from build123d import *

# Parameters (mm, degrees)
SKETCH1_W           = 70
SKETCH1_H           = 80
SKETCH1_R           = 17.5
SKETCH1_W_2         = 50
SKETCH1_H_2         = 30
BOSS_EXTRUDE1_DEPTH = 10
FILLET1_R           = 20
SKETCH2_R           = 2
CUT_EXTRUDE1_DEPTH  = 10


with BuildPart() as part:
    # Sketch1 → Boss-Extrude1 (new body)
    with BuildSketch(Plane.XY):
        with Locations((35, -40)):
            Rectangle(SKETCH1_W, SKETCH1_H)
        with Locations((35, -40)):
            Circle(SKETCH1_R, mode=Mode.SUBTRACT)
        with Locations((35, -95)):
            Rectangle(SKETCH1_W_2, SKETCH1_H_2)
    extrude(amount=BOSS_EXTRUDE1_DEPTH)

    # Fillet1
    fillet1_edges = [part.edges().sort_by_distance(p)[0] for p in [
        (70, 0, 5),
        (0, 0, 5),
    ]]
    fillet(fillet1_edges, radius=FILLET1_R)

    # Sketch2 → Cut-Extrude1 (cut)
    with BuildSketch(Plane.XY.offset(10)):
        with Locations((17.5, -22.5)):
            Circle(SKETCH2_R)
        with Locations((52.5, -22.5)):
            Circle(SKETCH2_R)
        with Locations((52.5, -57.5)):
            Circle(SKETCH2_R)
        with Locations((17.5, -57.5)):
            Circle(SKETCH2_R)
    extrude(amount=-CUT_EXTRUDE1_DEPTH, mode=Mode.SUBTRACT)


solid = part.part
CAD build for the part. Positions are in the model's coordinates, mm. A direction names the side the tool comes from. Round coordinates to 2 decimals unless told otherwise and drop trailing zeros. Write each loop counter-clockwise with the first axis right and the second up, starting at its lowest first coordinate (ties: lowest second). Pieces come first, ordered by that corner, then holes.
(1) 3-axis set-ups, long thin cutter, end or side, ignore diameter. For faces 5 (the face through (5, -80, 5)), 6 (the face through (52.24, -20.517, 5.07)), 7 (the face through (60, -95, 5)): which of +Z, -Z, +X, -X, +Y, -Y reach the whole face in a straight line?
(2) Slice it at D-D, the plane x = 62. Write the cut outline in (y, z).
(3) Mould opens along X. For faces 1 (the face through (17.24, -20.517, 5.07)), 2 (the face through (10, -95, 5)), 3 (the face through (64.297, -6.014, 5.07)), 4 (the face through (17.24, -55.517, 5.07)) say: pulls with the +X half, pulls with the -X half, needs draft (parallel to the pull), parting line crosses it, or undercut.
(4) Drop flat-ended pins along their axis: P1, Ø3.5, axis at x = 52.5, y = -22.5, coming from the -Z side; P2, Ø3, axis at x = 63.5, z = 3, coming from the -Y side. Give the stop position or say it passes through.
(5) Slice it at C-C, the plane z = 5.25. Write the cut outline in (x, y), and give its area (3 significant figures).
(6) Probe line 1 along Y through (x, z) = (35, 2.25); line 2 along Y through (x, z) = (47, 9.5); line 3 along X through (y, z) = (-101, 7.25). List the from-to ranges inside material, lowest first.
(7) Slice it at A-A, the plane x = 35. Write the cut outline in (y, z), and give its area (3 significant figures).
(8) Slice it at B-B, the plane y = -40. Write the cut outline in (x, z), and give its area (3 significant figures).
From the geometry:
1. face 5: +Z, -Z, -X, -Y
1. face 6: +Z, -Z
1. face 7: +Z, -Z, +X, -Y
2. outline: (-80, 0) - (-4, 0) - (-4, 10) - (-80, 10) - close
3. face 1: undercut
3. face 2: pulls with the -X half
3. face 3: pulls with the +X half
3. face 4: undercut
4. P1: passes through
4. P2: stops at y = -80
5. outline: (0, -80) - (10, -80) - (10, -110) - (60, -110) - (60, -80) - (70, -80) - (70, -20) arc R20 ccw to (50, 0) - (20, 0) arc R20 ccw to (0, -20) - close; hole circle Ø4 at (17.5, -57.5); hole circle Ø4 at (17.5, -22.5); hole circle Ø35 at (35, -40); hole circle Ø4 at (52.5, -57.5); hole circle Ø4 at (52.5, -22.5)
5. area: 5,920 mm2
6. line 1: y = -110 to -57.5, -22.5 to 0
6. line 2: y = -110 to -52.74, -27.26 to 0
6. line 3: x = 10 to 60
7. outline: (-110, 0) - (-57.5, 0) - (-57.5, 10) - (-110, 10) - close; (-22.5, 0) - (0, 0) - (0, 10) - (-22.5, 10) - close
7. area: 750 mm2
8. outline: (0, 0) - (17.5, 0) - (17.5, 10) - (0, 10) - close; (52.5, 0) - (70, 0) - (70, 10) - (52.5, 10) - close
8. area: 350 mm2
